Autodesk Inventor part; units mm, degrees
ref_plane "YZ Plane" through (0, 0, 0) normal (1, 0, 0) x (0, 1, 0)
ref_plane "XZ Plane" through (0, 0, 0) normal (0, 1, 0) x (-1, 0, 0)
ref_plane "XY Plane" through (0, 0, 0) normal (0, 0, 1) x (1, 0, 0)
sketch "Sketch1" plane through (0, 0, 0) normal (1, 0, 0) x (0, 1, 0)
  line L0 (0, 0) -> (66.04, 0)
  line L1 (66.04, 0) -> (66.04, -81.915)
  line L2 (66.04, -81.915) -> (0, -81.915)
  line L3 (0, -81.915) -> (0, 0)
  dimension "d0" = 66.04
  dimension "d1" = 81.915
extrude "Extrusion1" add sketch "Sketch1" along normal blind 31.75
fillet "Fillet1" radius 3.175 4 edges at (15.875, 0, -81.915) (15.875, 66.04, -81.915) (15.875, 0, 0) (15.875, 66.04, 0)
sketch "Sketch2" plane through (31.75, 0, 0) normal (1, 0, 0) x (0, 0, -1)
  line L0 (77.1525, 4.7625) -> (4.7625, 4.7625)
  line L1 (4.7625, 4.7625) -> (4.7625, 61.2775)
  line L2 (4.7625, 61.2775) -> (77.1525, 61.2775)
  line L3 (77.1525, 61.2775) -> (77.1525, 4.7625)
  line L4 (0, 0) -> (20.3539, 0) construction
  line L5 (3.175, 0) -> (78.74, 0)
  line L6 (0, 0) -> (0, 12.4806) construction
  line L7 (0, 62.865) -> (0, 3.175)
  dimension "d6" = 56.515
  dimension "d7" = 72.39
  dimension "d10" = 4.7625
  dimension "d19" = 4.7625
extrude "Extrusion2" cut sketch "Sketch2" against normal blind 12.7
sketch "Sketch3" plane through (19.05, 0, 0) normal (1, 0, 0) x (0, 0, -1)
  line L0 (77.1525, 61.2775) -> (77.1525, 4.7625)
  line L1 (77.1525, 33.02) -> (4.7625, 33.02) construction
  line L2 (4.7625, 4.7625) -> (4.7625, 61.2775)
  line L3 (4.7625, 7.62) -> (77.1525, 7.62)
  line L4 (77.1525, 7.62) -> (77.1525, 58.42)
  line L5 (77.1525, 58.42) -> (4.7625, 58.42)
  line L6 (4.7625, 58.42) -> (4.7625, 7.62)
  line L7 (4.7625, 7.62) -> (77.1525, 58.42) construction
  line L8 (77.1525, 7.62) -> (4.7625, 58.42) construction
  line L9 (77.1525, 4.7625) -> (4.7625, 4.7625)
  line L10 (77.1525, 4.7625) -> (77.1525, 24.7395)
  point P0 (40.9575, 33.02)
  dimension "d11" = 50.8
  dimension "d12" = 72.39
extrude "Extrusion3" cut sketch "Sketch3" against normal blind 13.208 contours L0 L3 L2 L5
fillet "Fillet3" radius 3.175 8 edges at (0, 0.9299, -80.9851) (0, 0, -40.9575) (0, 0.9299, -0.9299) (0, 33.02, 0) (0, 65.1101, -0.9299) (0, 66.04, -40.9575) (0, 65.1101, -80.9851) (0, 33.02, -81.915)
sketch "Sketch4" plane through (31.75, 0, 0) normal (1, 0, 0) x (0, 0, -1)
  line L0 (2.3813, -0.2223) -> (2.3813, 65.5235) construction
  line L1 (0, 3.175) -> (0, 62.865)
  circle A0 centre (2.3813, 7.62) radius 1.632
  line L2 (0, 62.865) -> (0, 3.175)
  line L3 (0, 33.02) -> (4.7625, 33.02) construction
  line L4 (4.7625, 7.62) -> (4.7625, 58.42)
  circle A1 centre (2.3812, 58.42) radius 1.632
  line L5 (4.7625, 58.42) -> (4.7625, 7.62)
  line L6 (77.1525, 4.7625) -> (4.7625, 4.7625)
  line L7 (40.9575, 4.7625) -> (40.9575, -0.2223) construction
  circle A2 centre (79.5338, 7.62) radius 1.632
  circle A3 centre (79.5338, 58.42) radius 1.632
  point P0 (0, 0)
  dimension "d17" = 2.3813
  dimension "d18" = 3.2639
  dimension "d21" = 25.4
extrude "Extrusion4" cut sketch "Sketch4" against normal blind 31.75
properties part number "bottom"
Input: part model. Units: mm. Frame: model coordinates. A direction names the side the tool comes from. Give positions to 0.01 mm unless a question says otherwise; leave off trailing zeros.
1. Set-up query: faces 4 (the face through (19.05, 6, -40)), 5 (the face through (0.91, 65.09, -41.49)). Return all of +Z, -Z, +X, -X, +Y, -Y with unobstructed straight access to the full face (end or side cutting, diameter ignored); none if empty.
Computed:
face 4: +X
face 5: +Z, -Z, -X, +Y
2. Line query: probe 1 along Z at (x, y) = (24.5, 58.42) (1 decimal); probe 2 along Z at (x, y) = (22, 18) (1 decimal); probe 3 along Y at (x, z) = (30, -61). Output: solid intervals per line, ascending.
Computed:
probe 1: z = -81.9 to -81.2, -77.9 to -77.2, -4.8 to -4, -0.7 to 0
probe 2: z = -81.9 to -77.2, -4.8 to 0
probe 3: y = 0 to 4.76, 61.28 to 66.04
3. Draft query along Z for faces 1 (the face through (0, 33, -40)), 2 (the face through (17, 33, 0)), 3 (the face through (16.097, 6.027, -2.028)). Return one class per face: released by +Z, released by -Z, zero draft, split by the parting line, or undercut.
Computed:
face 1: zero draft
face 2: released by +Z
face 3: undercut
4. Cut plane A-A (x = 22). State how many separate pieces and enclosed holes the cut face has, and give its area (3 significant figures).
Computed:
separate pieces: 1
enclosed holes: 5
area: 1,280 mm2
5. Pin query (flat end, axial travel): pin 1 Ø15 at (y, z) = (22.5, -54.5) entering from +X; pin 2 Ø2 at (y, z) = (7.62, -2.38) entering from -X; pin 3 Ø3 at (y, z) = (59.5, -36) entering from +X. Return the tip coordinate at first contact, or that it passes through.
Computed:
pin 1: stops at x = 5.84
pin 2: passes through
pin 3: stops at x = 19.05
